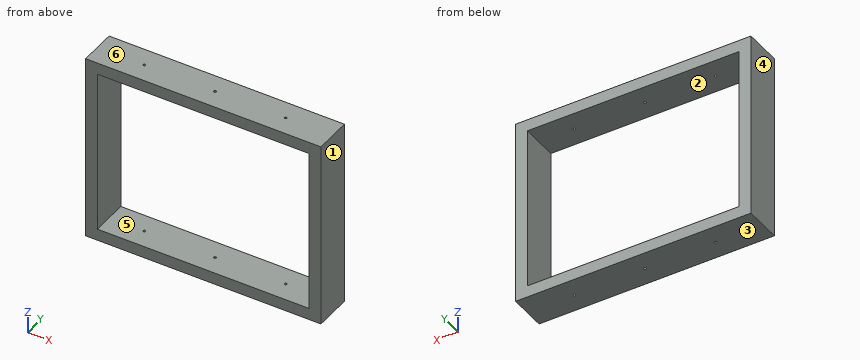
from build123d import *

# Parameters (mm, degrees)
F0_W     = 500
F0_H     = 400
F1_DEPTH = 80
F2_W     = 450
F2_H     = 350
F3_DEPTH = 80
F4_R     = 2.5
F5_DEPTH = 400.001


with BuildPart() as f1:
    # F0 (on Front) → F1 (new body)
    with BuildSketch(Plane.XZ):
        Rectangle(F0_W, F0_H)
    extrude(amount=F1_DEPTH)

    # F2 (on face) → F3 (cut, through all)
    with BuildSketch(Plane.XZ.offset(80)):
        Rectangle(F2_W, F2_H)
    extrude(amount=-F3_DEPTH, mode=Mode.SUBTRACT)

    # F4 (on face) → F5 (cut, through all)
    with BuildSketch(Plane.XY.offset(200)):
        with Locations((-150, -40)):
            Circle(F4_R)
        with Locations((0, -40)):
            Circle(F4_R)
        with Locations((150, -40)):
            Circle(F4_R)
    extrude(amount=-F5_DEPTH, mode=Mode.SUBTRACT)


solid = f1.part
Source: CAD feature listing. Evaluate the final solid. Frame: model axes, mm. Face numbers are marked on the shaded views. A direction names the side the tool comes from. Coordinates: 2 decimals unless noted, no trailing zeros. Order: outer loops, then holes, each group sorted by start corner. A loop starts at its lowest first (then second) coordinate and runs counter-clockwise, first axis right, second up. Notation, with made-up numbers: M -10,-38.5 L -3,-38.5 A15 cw -3,-20.5 Z; hole C 44.25,88 d9. An arc over 180 degrees is marked long. Write each question's results on one line, items separated by ' | '. Start each with the question number.
Item 1: Set-up query: the marked faces 1 and 2. Return all of +Z, -Z, +X, -X, +Y, -Y with unobstructed straight access to the full face (end or side cutting, diameter ignored); none if empty.
Item 2: Cut plane B-B (z = -4.5). Return loops of the section in (x, y), and give its area (3 significant figures).
Item 3: Draft query along Z for the marked faces 3, 4, 5 and 6. Return one class per face: pulls with the +Z half, pulls with the -Z half, needs draft (parallel to the pull), parting line crosses it, or undercut.
Item 4: Cut plane A-A (x = 94). Return loops of the section in (y, z), and give its area (3 significant figures).
Item 5: Line query: probe 1 along Z at (x, y) = (-125, -16.5); probe 2 along Y at (x, z) = (0, -184); probe 3 along X at (y, z) = (-35.5, 37). Output: solid intervals per line, ascending.
Item 6: Cut plane C-C (y = -58). Return loops of the section in (x, z).
Item 7: First-contact query: pin 1 Ø3 at (x, y) = (150, -40) entering from -Z. Flat tip, straight axial feed; report the tip coordinate or a pass-through.
Checked values:
1) face 1: +Z, -Z, +X, +Y, -Y | face 2: +Y, -Y
2) outline: M -250,-80 L -225,-80 L -225,0 L -250,0 Z; M 225,-80 L 250,-80 L 250,0 L 225,0 Z | area: 4,000 mm2
3) face 3: pulls with the -Z half | face 4: needs draft | face 5: undercut | face 6: pulls with the +Z half
4) outline: M -80,-200 L 0,-200 L 0,-175 L -80,-175 Z; M -80,175 L 0,175 L 0,200 L -80,200 Z | area: 4,000 mm2
5) probe 1: z = -200 to -175, 175 to 200 | probe 2: y = -80 to -42.5, -37.5 to 0 | probe 3: x = -250 to -225, 225 to 250
6) outline: M -250,-200 L 250,-200 L 250,200 L -250,200 Z; hole M -225,-175 L 225,-175 L 225,175 L -225,175 Z
7) pin 1: passes through
